Geometry check sheet. Reference: the model listing, model coordinates, mm. A direction names the side the tool comes from. Give positions to 0.01 mm unless a question says otherwise; leave off trailing zeros. Write each loop counter-clockwise with the first axis right and the second up, starting at its lowest first coordinate (ties: lowest second). Pieces come first, ordered by that corner, then holes. Notation, with made-up numbers: (22.25, -19) -> (75.25, -19) arc R10 cw to (75.25, -8) -> close; hole circle Ø7 at (85, 87.25). An arc over 180 degrees is marked (long way). Use a Markdown table: item, result. Add a question column.
from build123d import *

# Parameters (mm, degrees)
F1_DEPTH = 2.38
F2_R     = 2.465
F3_DEPTH = 25


with BuildPart() as f1:
    # F0 (on Top) → F1 (new body)
    with BuildSketch(Plane.XY):
        Polygon((-17.67767, 17.67767), (0, 0), (-10.355339, 25), (-15.202796, 20.152543), align=None)
        Polygon((0, 25), (0, 0), (10.355339, 25), (3.5, 25), align=None)
        Polygon((-10.355339, 25), (0, 0), (0, 25), (-3.5, 25), align=None)
        Polygon((-25, 10.355339), (0, 0), (-17.67767, 17.67767), (-20.152543, 15.202796), align=None)
        Polygon((-25, 0), (0, 0), (-25, 10.355339), (-25, 3.5), align=None)
        Polygon((-25, -10.355339), (0, 0), (-25, 0), (-25, -3.5), align=None)
        Polygon((-17.67767, -17.67767), (0, 0), (-25, -10.355339), (-20.152543, -15.202796), align=None)
        Polygon((-10.355339, -25), (0, 0), (-17.67767, -17.67767), (-15.202796, -20.152543), align=None)
        Polygon((0, -25), (0, 0), (-10.355339, -25), (-3.5, -25), align=None)
        Polygon((10.355339, -25), (0, 0), (0, -25), (3.5, -25), align=None)
        Polygon((17.67767, -17.67767), (0, 0), (10.355339, -25), (15.202796, -20.152543), align=None)
        Polygon((25, -10.355339), (0, 0), (17.67767, -17.67767), (20.152543, -15.202796), align=None)
        Polygon((25, 0), (0, 0), (25, -10.355339), (25, -3.5), align=None)
        Polygon((25, 10.355339), (0, 0), (25, 0), (25, 3.5), align=None)
        Polygon((17.67767, 17.67767), (0, 0), (25, 10.355339), (20.152543, 15.202796), align=None)
        Polygon((10.355339, 25), (0, 0), (17.67767, 17.67767), (15.202796, 20.152543), align=None)
        Polygon((-3.5, 25), (0, 25), (3.5, 25), (3.5, 28), (-3.5, 28), align=None)
        Polygon((-20.152543, 15.202796), (-17.67767, 17.67767), (-15.202796, 20.152543), (-17.324116, 22.273864), (-22.273864, 17.324116), align=None)
        Polygon((-25, -3.5), (-25, 0), (-25, 3.5), (-28, 3.5), (-28, -3.5), align=None)
        Polygon((-15.202796, -20.152543), (-17.67767, -17.67767), (-20.152543, -15.202796), (-22.273864, -17.324116), (-17.324116, -22.273864), align=None)
        Polygon((3.5, -25), (0, -25), (-3.5, -25), (-3.5, -28), (3.5, -28), align=None)
        Polygon((20.152543, -15.202796), (17.67767, -17.67767), (15.202796, -20.152543), (17.324116, -22.273864), (22.273864, -17.324116), align=None)
        Polygon((25, 3.5), (25, 0), (25, -3.5), (28, -3.5), (28, 3.5), align=None)
        Polygon((15.202796, 20.152543), (17.67767, 17.67767), (20.152543, 15.202796), (22.273864, 17.324116), (17.324116, 22.273864), align=None)
        Polygon((-8.5, 31.91786), (-3.5, 28), (3.5, 28), align=None)
        Polygon((-22.273864, 17.324116), (-17.324116, 22.273864), (-28.579743, 16.558928), align=None)
        Polygon((16.558928, 28.579743), (17.324116, 22.273864), (22.273864, 17.324116), align=None)
        Polygon((-28, -3.5), (-28, 3.5), (-31.91786, -8.5), align=None)
        Polygon((-17.324116, -22.273864), (-22.273864, -17.324116), (-16.558928, -28.579743), align=None)
        Polygon((3.5, -28), (-3.5, -28), (8.5, -31.91786), align=None)
        Polygon((22.273864, -17.324116), (17.324116, -22.273864), (28.579743, -16.558928), align=None)
        Polygon((28, 3.5), (28, -3.5), (31.91786, 8.5), align=None)
    extrude(amount=F1_DEPTH)

    # F2 (on face) → F3 (cut)
    with BuildSketch(Plane.XY.offset(2.38)):
        Circle(F2_R)
    extrude(amount=-F3_DEPTH, mode=Mode.SUBTRACT)


solid = f1.part
1) Sectioned sample at A-A, the plane x = 0. Enter the section's corners in (y, z) (3 decimals).
2) Gauge pin test, flat ends, axial feed: P1, Ø0.7, axis at y = -5.5, z = 0.5, coming from the +X side; P2, Ø1, axis at y = 6, z = 1, coming from the +X side; P3, Ø1.2, axis at x = -6.5, z = 1.5, coming from the -Y side. Record the tip position at first contact, or that the pin passes through.
3) Tool access check on faces 1 (the face through (-16.936, -25.471, 1.173)), 2 (the face through (25, -7, 1)), 3 (the face through (12.813, 22.542, 1.173)), 4 (the face through (-7, 25, 1)). Record the directions out of +Z, -Z, +X, -X, +Y, -Y that give a thin tool (end or side, any length) a straight path to the whole face; none if there is none.
4) Sectioned sample at C-C, the plane y = -9.5. Enter the section's corners in (x, z), and give its area (3 significant figures).
5) Draft check along Y on faces 5 (the face through (-22.87, 19.46, 1.17)), 6 (the face through (-1.956, -1.5, 1.207)), 7 (the face through (-26, 3.5, 1)), 8 (the face through (12.745, -22.61, 1.173)). Enter one of: +Y half, -Y half, draft (parallel to the pull), parting line (faces both ways), or undercut.
6) Material ranges on probe 1 along Y at (x, z) = (-20.5, 1.65); probe 2 along X at (y, z) = (-26.5, 2.2); probe 3 along X at (y, z) = (-6.5, 0.8), recorded low to high. Write a range as [from, to].
Check values:
| question | item | result |
|---|---|---|
| 1 | outline | (-29.143, 0) -> (-2.465, 0) -> (-2.465, 2.38) -> (-29.143, 2.38) -> close; (2.465, 0) -> (29.143, 0) -> (29.143, 2.38) -> (2.465, 2.38) -> close |
| 2 | P1 | x = 25 |
| 2 | P2 | x = 31.26 |
| 2 | P3 | y = -25 |
| 3 | face 1 | +Z, -Z |
| 3 | face 2 | +Z, -Z, +X |
| 3 | face 3 | +Z, -Z, +Y |
| 3 | face 4 | +Z, -Z, -X |
| 4 | outline | (-25, 0) -> (25, 0) -> (25, 2.38) -> (-25, 2.38) -> close |
| 4 | area | 119 mm² |
| 5 | face 5 | +Y half |
| 5 | face 6 | undercut |
| 5 | face 7 | undercut |
| 5 | face 8 | -Y half |
| 6 | probe 1 | [-20.82, -15.55], [-14.86, 14.86], [15.55, 20.66] |
| 6 | probe 2 | [-17.61, -16.81], [-3.5, 3.5] |
| 6 | probe 3 | [-31.26, -30.35], [-25, 25] |
